Input: part model. Units: mm. Frame: model coordinates. A direction names the side the tool comes from. Coordinates: 2 decimals unless noted, no trailing zeros. Order: outer loops, then holes, each group sorted by start corner. A loop starts at its lowest first (then second) coordinate and runs counter-clockwise, first axis right, second up. Notation, with made-up numbers: M 0.25,33 L 53.25,33 A9 ccw 53.25,41 Z; hole C -30.75,28.25 d2. An arc over 180 degrees is marked long. Answer in a Markdown table with one row per item.
from build123d import *

# Parameters (mm, degrees)
SKETCH1_R           = 25
BOSS_EXTRUDE1_DEPTH = 10
SKETCH2_R           = 3
CUT_EXTRUDE1_DEPTH  = 11


with BuildPart() as part:
    # Sketch1 → Boss-Extrude1 (new body)
    with BuildSketch(Plane.XY):
        Circle(SKETCH1_R)
        with BuildLine():
            Line((-4.472135955, -4), (4.472135955, -4))
            ThreePointArc((4.472135955, -4), (0, 6), (-4.472135955, -4))
        make_face(mode=Mode.SUBTRACT)
    extrude(amount=-BOSS_EXTRUDE1_DEPTH)

    # Sketch2 → Cut-Extrude1 (cut, through all)
    with BuildSketch(Plane(origin=(0, 0, -10), x_dir=(-1, 0, 0), z_dir=(0, 0, -1))):
        with Locations((0, 20)):
            Circle(SKETCH2_R)
        with Locations((17.320508076, -10)):
            Circle(SKETCH2_R)
        with Locations((-17.320508076, -10)):
            Circle(SKETCH2_R)
    extrude(amount=-CUT_EXTRUDE1_DEPTH, mode=Mode.SUBTRACT)


solid = part.part
1) Cut plane C-C, the plane z = -4. Output: boundary loops of the cut face in (x, y), and give its area (3 significant figures).
Resolved:
| item | result |
|---|---|
| outline | C 0,0 d50; hole C -17.32,-10 d6; hole M -4.47,-4 L 4.47,-4 A6 ccw long Z; hole C 0,20 d6; hole C 17.32,-10 d6 |
| area | 1,780 mm2 |
2) Mould query, pull axis Y, two halves, no side actions, for faces 1 (the face through (0, -5, -10)), 2 (the face through (23.846, 7.509, -4.93)), 3 (the face through (0.65, 17.07, -5.07)). Classes: +Y half, -Y half, draft (parallel to the pull), parting line (faces both ways), or undercut.
Resolved:
| item | result |
|---|---|
| face 1 | draft |
| face 2 | parting line |
| face 3 | undercut |
3) Reachability of faces 4 (the face through (0, -4, -5)), 5 (the face through (0, -5, 0)) from +Z, -Z, +X, -X, +Y, -Y: full face, straight path, thin tool, end or side. Return the list, or none.
Resolved:
| item | result |
|---|---|
| face 4 | +Z, -Z |
| face 5 | +Z, +X, -X, +Y, -Y |
4) Contact query for flat-ended pins moving along their axis: pin 1 (2 mm diameter, centred on y = 11, z = -1.5, fed in from -X); pin 2 (2 mm diameter, centred on x = -12.5, z = -6, fed in from -Y); pin 3 (6 mm diameter, centred on x = -10.5, z = -9, fed in from +Y); pin 4 (5 mm diameter, centred on x = 17.32, y = -10, fed in from +Z). Output: stop coordinate, or through.
Resolved:
| item | result |
|---|---|
| pin 1 | stops at x = -22.91 |
| pin 2 | stops at y = -22.2 |
| pin 3 | stops at y = 23.85 |
| pin 4 | passes through |
5) Cut plane A-A, the plane x = 0. Output: boundary loops of the cut face in (y, z).
Resolved:
| item | result |
|---|---|
| outline | M -25,-10 L -4,-10 L -4,0 L -25,0 Z; M 6,-10 L 17,-10 L 17,0 L 6,0 Z; M 23,-10 L 25,-10 L 25,0 L 23,0 Z |
6) Material intervals for probe 1 along X at (y, z) = (-9, -7.5); probe 2 along Y at (x, z) = (-2, -2); probe 3 along X at (y, z) = (-11, -5.25), sorted ascending.
Resolved:
| item | result |
|---|---|
| probe 1 | x = -23.32 to -20.15, -14.49 to 14.49, 20.15 to 23.32 |
| probe 2 | y = -24.92 to -4, 5.66 to 17.76, 22.24 to 24.92 |
| probe 3 | x = -22.45 to -20.15, -14.49 to 14.49, 20.15 to 22.45 |
7) Cut plane D-D, the plane y = 0. Output: boundary loops of the cut face in (x, z), and give its area (3 significant figures).
Resolved:
| item | result |
|---|---|
| outline | M -25,-10 L -6,-10 L -6,0 L -25,0 Z; M 6,-10 L 25,-10 L 25,0 L 6,0 Z |
| area | 380 mm2 |
8) Cut plane B-B, the plane y = 20. Output: boundary loops of the cut face in (x, z).
Resolved:
| item | result |
|---|---|
| outline | M -15,-10 L -3,-10 L -3,0 L -15,0 Z; M 3,-10 L 15,-10 L 15,0 L 3,0 Z |
